```python
from build123d import *

# Parameters (mm, degrees)
SKETCH1_R           = 2.5
BOSS_EXTRUDE1_DEPTH = 2
SKETCH2_W           = 50
SKETCH2_H           = 52
SKETCH2_R           = 13.25
SKETCH2_R_2         = 2.05
BOSS_EXTRUDE2_DEPTH = 2
BOSS_EXTRUDE3_DEPTH = 2
BOSS_EXTRUDE4_DEPTH = 2
FILLET1_R           = 5


with BuildPart() as part:
    # Sketch1 → Boss-Extrude1 (new body)
    with BuildSketch(Plane(origin=(0, 0, 0), x_dir=(1, 0, 0), z_dir=(0, 1, 0))):
        Polygon((35, 40), (35, 10), (85, 10), (85, 40), (120, 40), (120, 0), (0, 0), (0, 40), align=None)
        with Locations(Location((10, 30, 0), (0, 0, 270))):
            Circle(SKETCH1_R, mode=Mode.SUBTRACT)
        with Locations(Location((10, 10, 0), (0, 0, 270))):
            Circle(SKETCH1_R, mode=Mode.SUBTRACT)
        with Locations(Location((110, 10, 0), (0, 0, 90))):
            Circle(SKETCH1_R, mode=Mode.SUBTRACT)
        with Locations(Location((110, 30, 0), (0, 0, 90))):
            Circle(SKETCH1_R, mode=Mode.SUBTRACT)
    extrude(amount=BOSS_EXTRUDE1_DEPTH)

    # Sketch2 → Boss-Extrude2 (add)
    with BuildSketch(Plane(origin=(0, 0, -10), x_dir=(-1, 0, 0), z_dir=(0, 0, -1))):
        with Locations((-60, 26)):
            Rectangle(SKETCH2_W, SKETCH2_H)
        with Locations((-60, 27)):
            Circle(SKETCH2_R, mode=Mode.SUBTRACT)
        with Locations((-60, 44.5)):
            Circle(SKETCH2_R_2, mode=Mode.SUBTRACT)
        with Locations((-42.5, 27)):
            Circle(SKETCH2_R_2, mode=Mode.SUBTRACT)
        with Locations((-60, 9.5)):
            Circle(SKETCH2_R_2, mode=Mode.SUBTRACT)
        with Locations((-77.5, 27)):
            Circle(SKETCH2_R_2, mode=Mode.SUBTRACT)
    extrude(amount=BOSS_EXTRUDE2_DEPTH)

    # Sketch3 → Boss-Extrude3 (add)
    with BuildSketch(Plane.ZY.offset(-35)):
        Polygon((-12, 52), (-40, 2), (-32, 2), (-10, 41.285714286), (-10, 52), align=None)
    extrude(amount=BOSS_EXTRUDE3_DEPTH)

    # Sketch4 → Boss-Extrude4 (add)
    with BuildSketch(Plane(origin=(85, 0, 0), x_dir=(0, 0, -1), z_dir=(1, 0, 0))):
        Polygon((10, 52), (10, 41.285714286), (32, 2), (40, 2), (12, 52), align=None)
    extrude(amount=BOSS_EXTRUDE4_DEPTH)

    # Fillet1
    fillet1_edges = [part.edges().sort_by_distance(p)[0] for p in [
        (0, 1, -40),
        (120, 1, -40),
        (120, 1, 0),
        (0, 1, 0),
    ]]
    fillet(fillet1_edges, radius=FILLET1_R)


solid = part.part
```
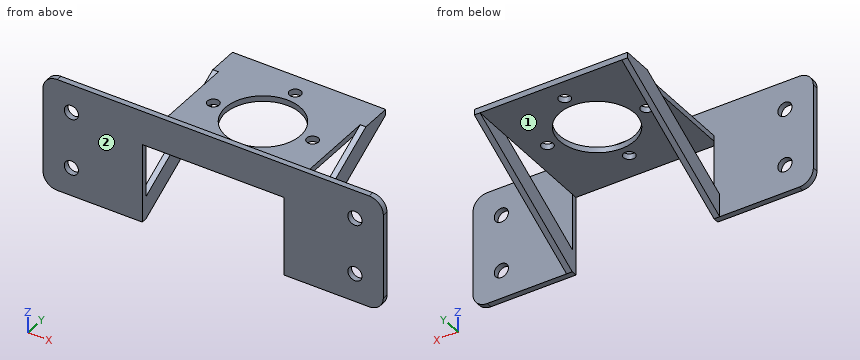
Geometry check sheet. Reference: the model listing, model coordinates, mm. Face numbers are marked on the shaded views. Coordinates: 2 decimals unless noted, no trailing zeros. Loops run counter-clockwise (first coordinate to the right, second up) from the corner with the lowest first, then second, coordinate; pieces in that order, holes last. Notation, with made-up numbers: (-8.5, 57) -> (40.5, 57) arc R23 cw to (40.5, 66) -> close; hole circle Ø8 at (-40, 57). An arc over 180 degrees is marked (long way). Put each result on its own line as item: value.
1) Cross-section at A-A on x = 10. Record the boundary of the cut face in (y, z).
Result set:
outline: (0, -40) -> (2, -40) -> (2, -32.5) -> (0, -32.5) -> close; (0, -27.5) -> (2, -27.5) -> (2, -12.5) -> (0, -12.5) -> close; (0, -7.5) -> (2, -7.5) -> (2, 0) -> (0, 0) -> close
2) Cross-section at B-B on y = 27. Record the boundary of the cut face in (x, z).
Result set:
outline: (33, -26) -> (35, -26) -> (35, -18) -> (33, -18) -> close; (35, -12) -> (40.45, -12) -> (40.45, -10) -> (35, -10) -> close; (44.55, -12) -> (46.75, -12) -> (46.75, -10) -> (44.55, -10) -> close; (73.25, -12) -> (75.45, -12) -> (75.45, -10) -> (73.25, -10) -> close; (79.55, -12) -> (85, -12) -> (85, -10) -> (79.55, -10) -> close; (85, -26) -> (87, -26) -> (87, -18) -> (85, -18) -> close
3) Cross-section at D-D on z = -30. Record the boundary of the cut face in (x, y), plus the area to 3 significant figures.
Result set:
outline: (0, 0) -> (7.5, 0) -> (7.5, 2) -> (0, 2) -> close; (12.5, 0) -> (35, 0) -> (35, 2) -> (12.5, 2) -> close; (33, 5.57) -> (35, 5.57) -> (35, 19.86) -> (33, 19.86) -> close; (85, 0) -> (107.5, 0) -> (107.5, 2) -> (85, 2) -> close; (85, 5.57) -> (87, 5.57) -> (87, 19.86) -> (85, 19.86) -> close; (112.5, 0) -> (120, 0) -> (120, 2) -> (112.5, 2) -> close
area: 177 mm^2
4) Release check for a two-part mould opening along X. For the marked faces 1 and 2 record: released by +X, released by -X, zero draft, split by the parting line, or undercut.
Result set:
face 1: undercut
face 2: zero draft
5) Thickness scan on line 1 (X direction, y = 19.5, z = -27); line 2 (Y direction, x = 60, z = -10.95); line 3 (Z direction, x = 46, y = 25). Record the ranges inside material, lowest first.
Result set:
line 1: x = 33 to 35, 85 to 87
line 2: y = 0 to 7.45, 11.55 to 13.75, 40.25 to 42.45, 46.55 to 52
line 3: z = -12 to -10
6) Gauge pin test, flat ends, axial feed: pin 1 Ø1.6 at (y, z) = (12.5, -11) entering from +X; pin 2 Ø24 at (y, z) = (26, -21.5) entering from -X; pin 3 Ø3.5 at (x, y) = (42.5, 27) entering from -Z; pin 4 Ø1 at (x, y) = (67.5, 10.5) entering from +Z. Record the tip position at first contact, or that the pin passes through.
Result set:
pin 1: stops at x = 85
pin 2: stops at x = 33
pin 3: passes through
pin 4: stops at z = -10
7) Cross-section at C-C on x = 60. Record the boundary of the cut face in (y, z).
Result set:
outline: (0, -12) -> (7.45, -12) -> (7.45, -10) -> (2, -10) -> (2, 0) -> (0, 0) -> close; (11.55, -12) -> (13.75, -12) -> (13.75, -10) -> (11.55, -10) -> close; (40.25, -12) -> (42.45, -12) -> (42.45, -10) -> (40.25, -10) -> close; (46.55, -12) -> (52, -12) -> (52, -10) -> (46.55, -10) -> close
